```python
from build123d import *

# Parameters (mm, degrees)
F0_R     = 18.522455
F1_DEPTH = 101.6
F3_W     = 85.290574
F3_H     = 49.032718
F4_DEPTH = 19.05
F2_W     = 84.098086
F2_H     = 49.134076
F5_DEPTH = 21.59
F6_R     = 12.7


with BuildPart() as f1:
    # F0 (on Right) → F1 (new body)
    with BuildSketch(Plane.YZ):
        Circle(F0_R)
    extrude(amount=F1_DEPTH)

    # F3 (on Front) → F4 (join)
    with BuildSketch(Plane.XZ):
        with Locations((-42.645287, 0)):
            Rectangle(F3_W, F3_H)
    extrude(amount=F4_DEPTH)

    # F2 (on Front) → F5 (join)
    with BuildSketch(Plane.XZ):
        with Locations((-42.049043, 0)):
            Rectangle(F2_W, F2_H)
    extrude(amount=-F5_DEPTH)

    # F6
    f6_edges = [f1.edges().sort_by_distance(p)[0] for p in [
        (-42.049043, 21.59, -24.567038),
        (-42.645287, -19.05, -24.516359),
    ]]
    fillet(f6_edges, radius=F6_R)


solid = f1.part
```
Design review of the part built by this model. Coordinates are the model's own, in mm. A direction names the side the tool comes from. Round coordinates to 2 decimals unless told otherwise and drop trailing zeros. Write each loop counter-clockwise with the first axis right and the second up, starting at its lowest first coordinate (ties: lowest second). Pieces come first, ordered by that corner, then holes.
Item 1: Clearance check with flat-ended pins moving along their axes: pin 1 Ø17.5 at (y, z) = (10.5, 1.5) entering from -X; pin 2 Ø1.5 at (x, y) = (74.5, 14) entering from +Z; pin 3 Ø1.5 at (x, z) = (30, 8.5) entering from -Y. State where each tip first meets the part, or that it passes through.
Item 2: For faces 1 (the cylindrical face through (-41.46, 17.968, -20.748)), 2 (the flat face through (-84.098, 11, 0)), 3 (the cylindrical face through (50.09, -14.7, -11.27)), list the 3-axis set-ups (+Z, -Z, +X, -X, +Y, -Y) from which the entire face can be reached by the end or side of a thin tool; tool diameter is ignored.
Item 3: For probe 1 along X at (y, z) = (14, -4); probe 2 along X at (y, z) = (13.5, 20.5); probe 3 along Y at (x, z) = (8, 12), list the stretches that pass through material, from the lowest coordinate up.
Item 4: We need section C-C on y = 16. Write out the cut boundary in (x, z).
Item 5: We need section B-B on x = -16. Write out the cut boundary in (y, z), and give its area (3 significant figures).
Item 6: We need section D-D on y = 3. Write out the cut boundary in (x, z), and give its area (3 significant figures).
Item 7: We need section A-A on z = 0. Write out the cut boundary in (x, y), and give its area (3 significant figures).
Returned:
1. pin 1: stops at x = -84.1
1. pin 2: stops at z = 12.94
1. pin 3: stops at y = -16.82
2. face 1: -Z, +X, -X, +Y
2. face 2: +Z, -Z, -X, +Y
2. face 3: +X
3. probe 1: x = -84.1 to 101.6
3. probe 2: x = -84.1 to 0
3. probe 3: y = -14.11 to 14.11
4. outline: (-84.1, -22.39) - (0, -22.39) - (0, -9.33) - (101.6, -9.33) - (101.6, 9.33) - (0, 9.33) - (0, 24.57) - (-84.1, 24.57) - close
5. outline: (-19.05, -11.82) arc R12.7 ccw to (-6.35, -24.52) - (0, -24.52) - (0, -24.57) - (8.89, -24.57) arc R12.7 ccw to (21.59, -11.87) - (21.59, 24.57) - (0, 24.57) - (0, 24.52) - (-19.05, 24.52) - close
5. area: 1,930 mm2
6. outline: (-84.1, -24.57) - (0, -24.57) - (0, -18.28) - (101.6, -18.28) - (101.6, 18.28) - (0, 18.28) - (0, 24.57) - (-84.1, 24.57) - close
6. area: 7,850 mm2
7. outline: (-85.29, -19.05) - (0, -19.05) - (0, -18.52) - (101.6, -18.52) - (101.6, 18.52) - (0, 18.52) - (0, 21.59) - (-84.1, 21.59) - (-84.1, 0) - (-85.29, 0) - close
7. area: 7,200 mm2
